Autodesk Inventor part; units mm, degrees
ref_plane "YZ Plane" through (0, 0, 0) normal (1, 0, 0) x (0, 1, 0)
ref_plane "XZ Plane" through (0, 0, 0) normal (0, 1, 0) x (-1, 0, 0)
ref_plane "XY Plane" through (0, 0, 0) normal (0, 0, 1) x (1, 0, 0)
sketch "Sketch1" plane through (0, 0, 0) normal (0, 1, 0) x (-1, 0, 0)
  line L0 (-75, 40) -> (75, 40)
  line L1 (75, 40) -> (75, -40)
  line L2 (75, -40) -> (-75, -40)
  line L3 (-75, -40) -> (-75, 40)
  line L4 (-75, 40) -> (75, -40) construction
  line L5 (75, 40) -> (-75, -40) construction
  point P0 (0, 0)
  dimension "d0" = 150
  dimension "d1" = 80
extrude "Extrusion1" add sketch "Sketch1" along normal blind 3
sketch "Sketch5" plane through (0, 3, 0) normal (0, 1, 0) x (1, 0, 0)
  line L0 (-75, 40) -> (-75, -40)
  line L1 (75, 40) -> (-75, 40)
  line L2 (-75, 40) -> (-75, 15)
  line L3 (-75, 15) -> (75, 15)
  line L4 (75, 15) -> (75, 40)
  line L5 (21.6, 15) -> (-21.6, 15)
  line L6 (75, 15) -> (31.8, 15)
  line L7 (31.8, 15) -> (31.8, -28.2)
  line L8 (31.8, -28.2) -> (75, -28.2)
  line L9 (75, -28.2) -> (75, 15)
  line L10 (31.8, 15) -> (75, -28.2)
  line L11 (75, 15) -> (31.8, -28.2)
  circle A0 centre (53.4, -6.6) radius 11
  line L12 (37.9, -22.1) -> (68.9, -22.1)
  line L13 (68.9, -22.1) -> (68.9, 8.9)
  line L14 (68.9, 8.9) -> (37.9, 8.9)
  line L15 (37.9, 8.9) -> (37.9, -22.1)
  line L16 (37.9, -22.1) -> (68.9, 8.9) construction
  line L17 (68.9, -22.1) -> (37.9, 8.9) construction
  circle A1 centre (37.9, 8.9) radius 2
  circle A2 centre (68.9, 8.9) radius 2
  circle A3 centre (68.9, -22.1) radius 2
  circle A4 centre (37.9, -22.1) radius 2
  point P0 (309.988, -32.2194)
  dimension "d26" = 25
  dimension "d49" = 150
  dimension "d50" = 43.2
  dimension "d51" = 43.2
  dimension "d52" = 22
  dimension "d53" = 31
  dimension "d54" = 31
  dimension "d55" = 4
  dimension "d56" = 4
  dimension "d57" = 4
  dimension "d58" = 4
extrude "Extrusion4" cut sketch "Sketch5" against normal through all contours A2 L13 L11 | L11 L14 A2 | A1 L14 L10 | L10 L15 A1 | A3 L12 L10 | L10 L13 A3 | L13 A2 L11 | L11 A2 L14 | A4 L15 L11 | L11 L12 A4 | L14 A1 L10 | L10 A1 L15 | L12 A3 L10 | L10 A3 L13 | L15 A4 L11 | L11 A4 L12 | A0 L10 L11 | L11 L10 A0 | L10 L11 A0 | A0 L11 L10
sketch "Sketch6" plane through (0, 3, 0) normal (0, 1, 0) x (1, 0, 0)
  line L0 (75, 40) -> (-75, 40)
  line L1 (0, 40) -> (0, 15)
  line L2 (0, 15) -> (0, -28.2)
  line L3 (-21.6, 15) -> (21.6, 15)
  line L4 (21.6, 15) -> (21.6, -28.2)
  line L5 (21.6, -28.2) -> (-21.6, -28.2)
  line L6 (-21.6, -28.2) -> (-21.6, 15)
  line L7 (-21.6, 15) -> (21.6, -28.2) construction
  line L8 (21.6, 15) -> (-21.6, -28.2) construction
  circle A0 centre (0, -6.6) radius 5.1
  line L9 (0, 15) -> (75, 15)
  line L10 (75, 15) -> (31.8, 15)
  line L11 (31.8, 15) -> (31.8, -6.6)
  line L12 (31.8, -6.6) -> (53.4, -6.6)
  line L13 (53.4, -6.6) -> (0, -6.6)
  line L14 (0, -6.6) -> (-53.4, -6.6)
  circle A1 centre (-53.4, -6.6) radius 4
  line L15 (0, -25.25) -> (0, 12.05)
  circle A2 centre (0, 12.05) radius 2.5
  line L16 (0, 12.05) -> (0, 10.05)
  circle A3 centre (0, 10.05) radius 2.5
  circle A4 centre (0, -25.25) radius 2.5
  line L17 (0, -25.25) -> (0, -23.25)
  circle A5 centre (0, -23.25) radius 2.5
  line L18 (-2.5, -23.25) -> (-2.5, -25.25)
  line L19 (2.5, -23.25) -> (2.5, -25.25)
  line L20 (-2.5, 12.05) -> (-2.5, 10.05)
  line L21 (2.5, 12.05) -> (2.5, 10.05)
  point P0 (0, 0)
  dimension "d59" = 25
  dimension "d60" = 43.2
  dimension "d61" = 43.2
  dimension "d62" = 43.2
  dimension "d63" = 10.2
  dimension "d64" = 43.2
  dimension "d65" = 53.4
  dimension "d66" = 8
  dimension "d69" = 37.3
  dimension "d70" = 5
  dimension "d71" = 2
  dimension "d72" = 5
  dimension "d73" = 5
  dimension "d74" = 2
  dimension "d75" = 5
extrude "Extrusion6" cut sketch "Sketch6" against normal through all contours L2 A3 A2 | L2 A2 A3 | A3 A2 L2 | L2 A2 A3 | A2 A3 L2 | L2 A3 A2 | A2 L21 A3 | A3 L20 A2 | A1 | A0 L13 L2 | L2 L14 A0 | L13 A0 L2 | L2 A0 L14 | A5 A4 L2 | L2 A4 A5 | A4 A5 L2 | L2 A5 A4 | L19 A4 A5 | A5 A4 L18 | A4 A5 L2 | L2 A5 A4
fillet "Fillet1" radius 20 4 edges at (75, 1.5, 40) (75, 1.5, -40) (-75, 1.5, 40) (-75, 1.5, -40)
properties part number "TopMount"
Verification items for the finished model (mm, model axes). A direction names the side the tool comes from. Give positions to 0.01 mm unless a question says otherwise; leave off trailing zeros. Order: outer loops, then holes, each group sorted by start corner. A loop starts at its lowest first (then second) coordinate and runs counter-clockwise, first axis right, second up. Notation, with made-up numbers: (-20, -39) -> (3, -39) arc R29 cw to (3, -13) -> close; hole circle Ø10 at (27, 74.25). An arc over 180 degrees is marked (long way). One line per item, written item: value.
(1) Sectioned sample at C-C on y = 0.7. Count the separate pieces of the cut face and the enclosed holes in it, then the cut area to 3 significant figures.
Final values:
separate pieces: 1
enclosed holes: 9
area: 11,000 mm^2
(2) Draft check along Z on faces 1 (the face through (-69.297, 1.521, 33.986)), 2 (the face through (66.902, 1.521, -8.988)), 3 (the face through (75, 1, 0)). Enter one of: pulls with the +Z half, pulls with the -Z half, needs draft (parallel to the pull), parting line crosses it, or undercut.
Final values:
face 1: pulls with the +Z half
face 2: undercut
face 3: needs draft
(3) Scan lines: line 1 along Z through (x, y) = (37.9, 1.35); line 2 along Z through (x, y) = (53.4, 2.1); line 3 along X through (y, z) = (1.1, -8.9). Record each from-to range of solid material in increasing order. Write a range as [from, to].
Final values:
line 1: [-40, -10.9], [-6.9, 20.1], [24.1, 40]
line 2: [-40, -4.4], [17.6, 40]
line 3: [-75, -2.22], [2.22, 35.9], [39.9, 66.9], [70.9, 75]
(4) Sectioned sample at B-B on z = 0. Record the cut outline in (x, y).
Final values:
outline: (-75, 0) -> (44.6, 0) -> (44.6, 3) -> (-75, 3) -> close; (62.2, 0) -> (75, 0) -> (75, 3) -> (62.2, 3) -> close
(5) Sectioned sample at D-D on x = 68.9. Record the cut outline in (y, z), then the cut area to 3 significant figures.
Final values:
outline: (0, -34.38) -> (3, -34.38) -> (3, -10.9) -> (0, -10.9) -> close; (0, -6.9) -> (3, -6.9) -> (3, 20.1) -> (0, 20.1) -> close; (0, 24.1) -> (3, 24.1) -> (3, 34.38) -> (0, 34.38) -> close
area: 182 mm^2
(6) Gauge pin test, flat ends, axial feed: pin 1 (0.6 mm diameter, centred on y = 2, z = 24.5, fed in from -X); pin 2 (3 mm diameter, centred on x = 37.9, z = 22.1, fed in from +Y). Record the tip position at first contact, or that the pin passes through.
Final values:
pin 1: x = -74.55
pin 2: through
(7) Sectioned sample at A-A on x = 53.4. Record the cut outline in (y, z).
Final values:
outline: (0, -40) -> (3, -40) -> (3, -4.4) -> (0, -4.4) -> close; (0, 17.6) -> (3, 17.6) -> (3, 40) -> (0, 40) -> close
(8) Tool access check on faces 4 (the face through (1, 3, 1)), 5 (the face through (0.05, 1.52, 20.75)). Record the directions out of +Z, -Z, +X, -X, +Y, -Y that give a thin tool (end or side, any length) a straight path to the whole face; none if there is none.
Final values:
face 4: +Z, -Z, +X, -X, +Y
face 5: +Y, -Y
